The model under review builds one solid part; all positions refer to its coordinate system, in mm. A direction names the side the tool comes from. Coordinates: 2 decimals unless noted, no trailing zeros. Loops run counter-clockwise (first coordinate to the right, second up) from the corner with the lowest first, then second, coordinate; pieces in that order, holes last. Notation, with made-up numbers: (-28, -39.75) - (-16, -39.75) arc R26 ccw to (-16, -10.75) - close; hole circle Ø10 at (73.5, 70). An arc over 180 degrees is marked (long way). Use a Markdown table: item, result. Add a question column.
1) Add section D-D, the plane x = 11. Give the boundary of the cut face in (y, z).
2) Add section B-B, the plane z = 2.45. Give the number of separate pieces and of enclosed holes in the cut face, and give its area (3 significant figures).
3) To check wall thickness, follow L1, parallel to Y at x = 20.5, z = 1.45; L2, parallel to X at y = 10, z = 1.2; L3, parallel to Y at x = -6, z = 2.05. State the ranges of each line that lie inside material, in increasing order. Write a range as [from, to].
4) Add section A-A, the plane x = 20.5. Give the boundary of the cut face in (y, z).
5) For faces 1 (the flat face through (-15.9, 11, 2)), 2 (the flat face through (-21, 0, 2)), 3 (the cylindrical face through (-29.658, -14.639, 1.014)), list the 3-axis set-ups (+Z, -Z, +X, -X, +Y, -Y) from which the entire face can be reached by the end or side of a thin tool; tool diameter is ignored.
6) Clearance check with flat-ended pins moving along their axes: pin 1 (13 mm diameter, centred on x = -0.5, y = 8.5, fed in from +Z); pin 2 (4 mm diameter, centred on x = -20.5, y = 10, fed in from -Z); pin 3 (2.5 mm diameter, centred on x = -20.5, y = -5, fed in from +Z); pin 4 (0.5 mm diameter, centred on y = 7, z = 2.5, fed in from +X). State where each tip first meets the part, or that it passes through.
7) The part is to be moulded in two halves that separate along Y. For faces 4 (the flat face through (20, 0, 2)), 5 (the flat face through (-11, 0, 1)), 6 (the cylindrical face through (29.639, -14.658, 1.014)), say which applies: pulls with the +Y half, pulls with the -Y half, needs draft (parallel to the pull), parting line crosses it, or undercut.
8) Add section C-C, the plane y = 2. Give the boundary of the cut face in (x, z).
Autodesk Inventor part; units mm, degrees
ref_plane "YZ Plane" through (0, 0, 0) normal (1, 0, 0) x (0, 1, 0)
ref_plane "XZ Plane" through (0, 0, 0) normal (0, 1, 0) x (-1, 0, 0)
ref_plane "XY Plane" through (0, 0, 0) normal (0, 0, 1) x (1, 0, 0)
sketch "スケッチ1" plane through (0, 0, 0) normal (0, 0, 1) x (1, 0, 0)
  line L0 (-30, -15) -> (30, -15)
  line L1 (30, -15) -> (30, 15)
  line L2 (30, 15) -> (-30, 15)
  line L3 (-30, 15) -> (-30, -15)
  line L4 (-30, -15) -> (30, 15) construction
  line L5 (30, -15) -> (-30, 15) construction
  point P0 (0, 0)
  dimension "d0" = 60
  dimension "d1" = 30
extrude "押し出し1" add sketch "スケッチ1" along normal blind 3
sketch "スケッチ2" plane through (0, 0, 3) normal (0, 0, 1) x (1, 0, 0)
  line L0 (30, 15) -> (-30, 15)
  line L1 (-30, -15) -> (30, -15)
  line L2 (-17.9, 15) -> (-23.1, 15)
  line L3 (-23.1, 15) -> (-23.1, -15)
  line L4 (-23.1, -15) -> (-17.9, -15)
  line L5 (-17.9, -15) -> (-17.9, 15)
  line L6 (17.9, -15) -> (23.1, -15)
  line L7 (23.1, -15) -> (23.1, 15)
  line L8 (23.1, 15) -> (17.9, 15)
  line L9 (17.9, 15) -> (17.9, -15)
  point P0 (0, 0)
  dimension "d4" = 5.2
  dimension "d5" = 5.2
  dimension "d6" = 17.9
  dimension "d7" = 17.9
extrude "押し出し2" cut sketch "スケッチ2" against normal blind 1 contours L7 L1 L9 L0 | L5 L1 L3 L0
sketch "スケッチ3" plane through (0, 0, 2) normal (0, 0, 1) x (1, 0, 0)
  line L0 (-23.1, 15) -> (-17.9, 15)
  line L1 (-17.9, -15) -> (-23.1, -15)
  line L2 (23.1, -15) -> (17.9, -15)
  line L3 (17.9, 15) -> (23.1, 15)
  line L4 (-20.5, 15) -> (-20.5, -15) construction
  line L5 (20.5, -15) -> (20.5, 15) construction
  point P0 (0, 0)
  point P1 (-20.5, 10)
  point P2 (-20.5, -10)
  point P3 (20.5, -10)
  point P4 (20.5, 10)
  dimension "d10" = 5
  dimension "d11" = 5
  dimension "d12" = 5
  dimension "d13" = 5
hole "穴1" at (-20.5, 10, 2) at (-20.5, -10, 2) at (20.5, -10, 2) at (20.5, 10, 2) direction (0, 0, -1) diameter 3.5 end through all
chamfer "面取り1" distance 1 angle 45 4 edges at (-20.5, -8.25, 0) (20.5, -8.25, 0) (-20.5, 11.75, 0) (20.5, 11.75, 0)
sketch "スケッチ4" plane through (0, 0, 3) normal (0, 0, 1) x (1, 0, 0)
  line L0 (17.9, -15) -> (17.9, 15)
  line L1 (17.9, 15) -> (-17.9, 15)
  line L2 (-17.9, 15) -> (-17.9, -15)
  line L3 (-17.9, -15) -> (17.9, -15)
  line L4 (-15.9, 13) -> (15.9, 13)
  line L5 (15.9, 13) -> (15.9, -13)
  line L6 (15.9, -13) -> (-15.9, -13)
  line L7 (-15.9, -13) -> (-15.9, 13)
  circle A0 centre (-20.5, 10) radius 1.75
  circle A1 centre (20.5, -10) radius 1.75
  circle A2 centre (20.5, 10) radius 1.75
  circle A3 centre (-20.5, -10) radius 1.75
  circle A4 centre (20.5, -10) radius 2.75 construction
  line L8 (-20.5, 10) -> (20.5, -10) construction
  line L9 (-20.5, -10) -> (20.5, 10) construction
  line L10 (-20.0616, -10.8988) -> (20.9384, 9.1012)
  line L11 (20.9384, 9.1012) -> (20.0616, 10.8988)
  line L12 (20.0616, 10.8988) -> (-20.9384, -9.1012)
  line L13 (-20.9384, -9.1012) -> (-20.0616, -10.8988)
  line L14 (-20.0616, -10.8988) -> (20.0616, 10.8988) construction
  line L15 (20.9384, 9.1012) -> (-20.9384, -9.1012) construction
  line L16 (20.0616, -10.8988) -> (-20.9384, 9.1012)
  line L17 (-20.9384, 9.1012) -> (-20.0616, 10.8988)
  line L18 (-20.0616, 10.8988) -> (20.9384, -9.1012)
  line L19 (20.9384, -9.1012) -> (20.0616, -10.8988)
  line L20 (20.0616, -10.8988) -> (-20.0616, 10.8988) construction
  line L21 (-20.9384, 9.1012) -> (20.9384, -9.1012) construction
  point P0 (0, 0)
  point P1 (15.9, -8.8687)
  point P2 (0, -1.1126)
  point P3 (-15.9, -8.8687)
  point P4 (2.2809, 0)
  point P5 (15.9, -6.6435)
  point P6 (15.9, 6.6435)
  point P7 (-2.2809, 0)
  point P8 (-15.9, 6.6435)
  point P9 (-15.9, -6.6435)
  point P10 (-15.9, 8.8687)
  point P11 (0, 1.1126)
  point P12 (15.9, 8.8687)
  dimension "d24" = 2
  dimension "d25" = 2
  dimension "d26" = 2
extrude "押し出し3" cut sketch "スケッチ4" against normal blind 2 contours L5 L6 L7 L10 L16 | L18 L10 L5 | L12 L7 L16 | L12 L18 L7 L4 L5
fillet "フィレット1" radius 1 16 edges at (-15.9, 6.6435, 2) (-15.9, -6.6435, 2) (-2.2809, 0, 2) (0, -1.1126, 2) (2.2809, 0, 2) (15.9, -6.6435, 2) (15.9, -8.8687, 2) (15.9, -13, 2) (-15.9, -13, 2) (-15.9, -8.8687, 2) (15.9, 6.6435, 2) (15.9, 8.8687, 2) (15.9, 13, 2) (-15.9, 13, 2) (-15.9, 8.8687, 2) (0, 1.1126, 2)
fillet "フィレット2" radius 1.2 4 edges at (-30, 15, 1.5) (-30, -15, 1.5) (30, -15, 1.5) (30, 15, 1.5)
chamfer "面取り2" distance 1 angle 45 10 edges at (-30, 0, 3) (-29.6485, -14.6485, 3) (-25.95, -15, 3) (-29.6485, 14.6485, 3) (-25.95, 15, 3) (30, 0, 3) (29.6485, 14.6485, 3) (25.95, 15, 3) (29.6485, -14.6485, 3) (25.95, -15, 3)
equation "\"d5\" = d4"
properties part number "3D_club_3D プリント"
From the geometry:
| question | item | result |
|---|---|---|
| 1 | outline | (-15, 0) - (15, 0) - (15, 3) - (13, 3) - (13, 1) - (6.48, 1) - (6.48, 3) - (4.25, 3) - (4.25, 1) - (-4.25, 1) - (-4.25, 3) - (-6.48, 3) - (-6.48, 1) - (-13, 1) - (-13, 3) - (-15, 3) - close |
| 2 | separate pieces | 3 |
| 2 | enclosed holes | 4 |
| 2 | area | 764 mm^2 |
| 3 | L1 | y = [-15, -11.75], [-8.25, 8.25], [11.75, 15] |
| 3 | L2 | x = [-30, -22.25], [-18.75, -15.9], [15.9, 18.75], [22.25, 30] |
| 3 | L3 | y = [-15, -13], [-4.04, -1.81], [1.81, 4.04], [13, 15] |
| 4 | outline | (-15, 0) - (-12.75, 0) - (-11.75, 1) - (-11.75, 2) - (-15, 2) - close; (-8.25, 1) - (-7.25, 0) - (7.25, 0) - (8.25, 1) - (8.25, 2) - (-8.25, 2) - close; (11.75, 1) - (12.75, 0) - (15, 0) - (15, 2) - (11.75, 2) - close |
| 5 | face 1 | +Z |
| 5 | face 2 | +Z, +Y, -Y |
| 5 | face 3 | +Z, -Z, -X, -Y |
| 6 | pin 1 | stops at z = 3 |
| 6 | pin 2 | stops at z = 0.75 |
| 6 | pin 3 | stops at z = 2 |
| 6 | pin 4 | stops at x = 29.75 |
| 7 | face 4 | needs draft |
| 7 | face 5 | undercut |
| 7 | face 6 | pulls with the -Y half |
| 8 | outline | (-30, 0) - (30, 0) - (30, 2) - (29, 3) - (23.1, 3) - (23.1, 2) - (17.9, 2) - (17.9, 3) - (15.9, 3) - (15.9, 1) - (6.38, 1) - (6.38, 3) - (1.82, 3) - (1.82, 1) - (-1.82, 1) - (-1.82, 3) - (-6.38, 3) - (-6.38, 1) - (-15.9, 1) - (-15.9, 3) - (-17.9, 3) - (-17.9, 2) - (-23.1, 2) - (-23.1, 3) - (-29, 3) - (-30, 2) - close |
